Model file for the job. Use its own axes, mm. A direction names the side the tool comes from. Round coordinates to 2 decimals unless told otherwise and drop trailing zeros. Order: outer loops, then holes, each group sorted by start corner. A loop starts at its lowest first (then second) coordinate and runs counter-clockwise, first axis right, second up. Notation, with made-up numbers: (-38.75, 84.25) -> (-29.75, 84.25) arc R37 ccw to (-29.75, 121.25) -> close; hole circle Ø2 at (-15, -16.5). An arc over 180 degrees is marked (long way). Answer as CSV lines item,"result".
Autodesk Inventor part; units mm, degrees
ref_plane "YZ Plane" through (0, 0, 0) normal (1, 0, 0) x (0, 1, 0)
ref_plane "XZ Plane" through (0, 0, 0) normal (0, 1, 0) x (-1, 0, 0)
ref_plane "XY Plane" through (0, 0, 0) normal (0, 0, 1) x (1, 0, 0)
sketch "Эскиз1" plane through (0, 0, 0) normal (0, 0, 1) x (1, 0, 0)
  line L0 (-150, 116) -> (150, 116)
  line L1 (165, 101) -> (165, -101)
  line L2 (150, -116) -> (-150, -116)
  line L3 (-165, -101) -> (-165, 101)
  line L4 (-252.8728, 0) -> (252.8728, 0)
  line L5 (0, -184.2728) -> (0, 184.2728)
  arc A0 (-150, 116) -> (-165, 101) centre (-150, 101) ccw
  arc A1 (165, 101) -> (150, 116) centre (150, 101) ccw
  arc A2 (150, -116) -> (165, -101) centre (150, -101) ccw
  arc A3 (-165, -101) -> (-150, -116) centre (-150, -101) ccw
  line L6 (-175.3693, 101) -> (-175.3693, -101)
  arc A4 (-175.3693, -101) -> (-150, -126.3693) centre (-150, -101) ccw
  line L7 (-150, -126.3693) -> (150, -126.3693)
  arc A5 (150, -126.3693) -> (175.3693, -101) centre (150, -101) ccw
  line L8 (175.3693, -101) -> (175.3693, 101)
  arc A6 (175.3693, 101) -> (150, 126.3693) centre (150, 101) ccw
  line L9 (150, 126.3693) -> (-150, 126.3693)
  arc A7 (-150, 126.3693) -> (-175.3693, 101) centre (-150, 101) ccw
  point P0 (0, 0)
  dimension "d0" = 232
  dimension "d1" = 330
  dimension "d2" = 15
extrude "Выдавливание1" add sketch "Эскиз1" along normal blind 110 contours A0 L3 L4 L6 A7 L9 L5 L0 | L5 L9 A6 L8 L4 L1 A1 L0 | L3 A3 L2 L5 L7 A4 L6 L4 | L4 L8 A5 L7 L5 L2 A2 L1
sketch "Эскиз2" plane through (0, 0, 0) normal (0, 0, -1) x (-1, 0, 0)
  line L0 (150, -126.3693) -> (-150, -126.3693)
  arc A0 (150, -126.3693) -> (175.3693, -101) centre (150, -101) ccw
  line L1 (175.3693, 101) -> (175.3693, -101)
  arc A1 (175.3693, 101) -> (150, 126.3693) centre (150, 101) ccw
  line L2 (-150, 126.3693) -> (150, 126.3693)
  arc A2 (-150, 126.3693) -> (-175.3693, 101) centre (-150, 101) ccw
  line L3 (-175.3693, -101) -> (-175.3693, 101)
  arc A3 (-175.3693, -101) -> (-150, -126.3693) centre (-150, -101) ccw
  point P0 (0, 0)
extrude "Выдавливание2" add sketch "Эскиз2" along normal blind 10
fillet "Сопряжение1" radius 15 8 edges at (-167.9388, -118.9388, -10) (-175.3693, 0, -10) (-167.9388, 118.9388, -10) (0, 126.3693, -10) (167.9388, 118.9388, -10) (175.3693, 0, -10) (167.9388, -118.9388, -10) (0, -126.3693, -10)
fillet "Сопряжение2" radius 15 8 edges at (160.6066, 111.6066, 0) (165, 0, 0) (160.6066, -111.6066, 0) (0, -116, 0) (-160.6066, -111.6066, 0) (-165, 0, 0) (-160.6066, 111.6066, 0) (0, 116, 0)
properties part number "Корпус НАСУ"
Q1. Mould opens along X. For faces 3 (the flat face through (2, 126.369, 58)), 4 (the cylindrical face through (-168.135, -118.74, 58.235)), 5 (the cylindrical face through (-2.1, 111.72, 4.51)) say: +X half, -X half, draft (parallel to the pull), parting line (faces both ways), or undercut.
Checks:
face 3,"draft"
face 4,"-X half"
face 5,"undercut"
Q2. Flat gauge pin, fed straight in: pin 1 (8 mm diameter, centred on x = -122.5, y = 68.5, fed in from +Z). Where does the tip first touch, or does it go through?
Checks:
pin 1,"z = 0"
Q3. Saw through at B-B (y = 72). Write the cut outline in (x, z), plus the area to 3 significant figures.
Checks:
outline,"(-175.37, 5) arc R15 ccw to (-160.37, -10) -> (160.37, -10) arc R15 ccw to (175.37, 5) -> (175.37, 110) -> (165, 110) -> (165, 15) arc R15 cw to (150, 0) -> (-150, 0) arc R15 cw to (-165, 15) -> (-165, 110) -> (-175.37, 110) -> close"
area,"5,790 mm²"
Q4. Tool access for faces 1 (the cylindrical face through (160.72, -111.49, 61.84)), 2 (the cylindrical face through (167.74, -119.135, 58.235)): list every direction of +Z, -Z, +X, -X, +Y, -Y with a clear straight run to the whole face (end or side of a thin tool).
Checks:
face 1,"+Z"
face 2,"+Z, -Z, +X, -Y"
Q5. Wall check: L1, parallel to Y at x = 5.5, z = 41; L2, parallel to X at y = 59.5, z = 72; L3, parallel to Z at x = -54, y = 11.5. Give the ranges that are in metal, low to high. Write a range as [from, to].
Checks:
L1,"[-126.37, -116], [116, 126.37]"
L2,"[-175.37, -165], [165, 175.37]"
L3,"[-10, 0]"
Q6. Saw through at A-A (z = 24.5). Write the cut outline in (x, y), plus the area to 3 significant figures.
Checks:
outline,"(-175.37, -101) arc R25.37 ccw to (-150, -126.37) -> (150, -126.37) arc R25.37 ccw to (175.37, -101) -> (175.37, 101) arc R25.37 ccw to (150, 126.37) -> (-150, 126.37) arc R25.37 ccw to (-175.37, 101) -> close; hole (-165, -101) arc R15 ccw to (-150, -116) -> (150, -116) arc R15 ccw to (165, -101) -> (165, 101) arc R15 ccw to (150, 116) -> (-150, 116) arc R15 ccw to (-165, 101) -> close"
area,"11,700 mm²"
Q7. Saw through at C-C (x = -9.5). Write the cut outline in (y, z).
Checks:
outline,"(-126.37, 5) arc R15 ccw to (-111.37, -10) -> (111.37, -10) arc R15 ccw to (126.37, 5) -> (126.37, 110) -> (116, 110) -> (116, 15) arc R15 cw to (101, 0) -> (-101, 0) arc R15 cw to (-116, 15) -> (-116, 110) -> (-126.37, 110) -> close"
